Verification items for the finished model (mm, model axes). A direction names the side the tool comes from. Round coordinates to 2 decimals unless told otherwise and drop trailing zeros. Loops run counter-clockwise (first coordinate to the right, second up) from the corner with the lowest first, then second, coordinate; pieces in that order, holes last. Notation, with made-up numbers: (54, -22) -> (65, -22) arc R24 cw to (65, -3) -> close; hole circle Ø7 at (33.5, -25.5). An arc over 180 degrees is marked (long way). Write item = value, one per line. Start each with the question number.
Autodesk Inventor part; units mm, degrees
ref_plane "YZ Plane" through (0, 0, 0) normal (1, 0, 0) x (0, 1, 0)
ref_plane "XZ Plane" through (0, 0, 0) normal (0, 1, 0) x (-1, 0, 0)
ref_plane "XY Plane" through (0, 0, 0) normal (0, 0, 1) x (1, 0, 0)
sketch "Sketch1" plane through (0, 0, 0) normal (0, 1, 0) x (-1, 0, 0)
  line L0 (0, 0) -> (15, 0)
  line L1 (15, 0) -> (15, -76.2)
  line L2 (15, -76.2) -> (0, -76.2)
  line L3 (0, -76.2) -> (0, 0)
  circle A0 centre (7.5, -12.7) radius 1.7
  circle A1 centre (7.5, -63.5) radius 1.7
  dimension "d0" = 15
  dimension "d1" = 76.2
  dimension "d2" = 3.4
  dimension "d3" = 3.4
  dimension "d4" = 12.7
  dimension "d5" = 12.7
extrude "Extrusion1" add sketch "Sketch1" along normal blind 12.3698
sketch "Sketch2" plane through (0, 12.3698, 0) normal (0, 1, 0) x (1, 0, 0)
  circle A0 centre (-7.5, 28.321) radius 1.9685 construction
  circle A1 centre (-7.5, 47.879) radius 1.9685 construction
  line L0 (-15, 76.2) -> (-15, 0)
  line L1 (0, 76.2) -> (-15, 76.2)
  line L2 (-15, 0) -> (0, 0)
  dimension "d8" = 3.937
  dimension "d9" = 3.937
  dimension "d10" = 19.558
  dimension "d11" = 7.5
  dimension "d12" = 7.5
  dimension "d13" = 28.321
  dimension "d14" = 28.321
hole "Hole1" at (-7.5, 12.3698, -28.321) at (-7.5, 12.3698, -47.879) direction (0, -1, 0) diameter 3.937 depth 20.32 counterbore diameter 5.969 counterbore depth 4.953
fillet "Fillet1" radius 3.175 4 edges at (-15, 6.1849, -76.2) (0, 6.1849, -76.2) (0, 6.1849, 0) (-15, 6.1849, 0)
properties part number "Collection rotation adapter"
(1) Section check B-B on z = -12.7. Enter the section's corners in (x, y), then the cut area to 3 significant figures.
(2) Depth check by flat-ended pin: pin 1 Ø3 at (x, z) = (-6.5, -27.5) entering from +Y. Enter the tip coordinate at first touch or a pass-through.
(3) Section check A-A on x = -7.5. Enter the section's corners in (y, z), then the cut area to 3 significant figures.
(4) Scan lines: line 1 (Z direction, x = -7.5, y = 6.75); line 2 (Z direction, x = -7.5, y = 9.65); line 3 (Z direction, x = -5.25, y = 8.5). Record each from-to range of solid material in increasing order. Write a range as [from, to].
(5) Section check C-C on y = 11.25. Give the number of separate pieces and of enclosed holes in the cut face, then the cut area to 3 significant figures.
(6) Draft check along Z on faces 1 (the flat face through (-7, 0, -38)), 2 (the cylindrical face through (-14.09, 6.27, -0.95)), 3 (the flat face through (-8, 7.417, -50)). Enter one of: +Z half, -Z half, draft (parallel to the pull), parting line (faces both ways), or undercut.
(7) Access from +Z, -Z, +X, -X, +Y, -Y to the whole of each face (thin tool, end or side, straight path). Record for faces 4 (the cylindrical face through (-7.631, 9.859, -31.303)), 5 (the flat face through (-7, 6, 0)).
Computed values:
q1.outline = (-15, 0) -> (-9.2, 0) -> (-9.2, 12.37) -> (-15, 12.37) -> close; (-5.8, 0) -> (0, 0) -> (0, 12.37) -> (-5.8, 12.37) -> close
q1.area = 143 mm²
q2.pin_1 = 7.42
q3.outline = (0, -76.2) -> (12.37, -76.2) -> (12.37, -65.2) -> (0, -65.2) -> close; (0, -61.8) -> (12.37, -61.8) -> (12.37, -50.86) -> (7.42, -50.86) -> (7.42, -49.85) -> (0, -49.85) -> close; (0, -45.91) -> (7.42, -45.91) -> (7.42, -44.89) -> (12.37, -44.89) -> (12.37, -31.31) -> (7.42, -31.31) -> (7.42, -30.29) -> (0, -30.29) -> close; (0, -26.35) -> (7.42, -26.35) -> (7.42, -25.34) -> (12.37, -25.34) -> (12.37, -14.4) -> (0, -14.4) -> close; (0, -11) -> (12.37, -11) -> (12.37, 0) -> (0, 0) -> close
q3.area = 741 mm²
q4.line_1 = [-76.2, -65.2], [-61.8, -49.85], [-45.91, -30.29], [-26.35, -14.4], [-11, 0]
q4.line_2 = [-76.2, -65.2], [-61.8, -50.86], [-44.89, -31.31], [-25.34, -14.4], [-11, 0]
q4.line_3 = [-76.2, -49.84], [-45.92, -30.28], [-26.36, 0]
q5.separate_pieces = 1
q5.enclosed_holes = 4
q5.area = 1,060 mm²
q6.face_1 = draft
q6.face_2 = +Z half
q6.face_3 = undercut
q7.face_4 = +Y
q7.face_5 = +Z, +X, -X, +Y, -Y
